The listing builds one solid part. Answer for the finished solid, in the listing's coordinates (mm). A direction names the side the tool comes from. Give positions to 0.01 mm unless a question says otherwise; leave off trailing zeros. Write each loop counter-clockwise with the first axis right and the second up, starting at its lowest first coordinate (ties: lowest second). Pieces come first, ordered by that corner, then holes. Notation, with made-up numbers: (17.25, -24.5) -> (48.25, -24.5) arc R18 cw to (48.25, -19.5) -> close; hole circle Ø9 at (77, 41). An arc over 180 degrees is marked (long way). Write each question's results on one line, items separated by ' | '. Start each with the question number.
from build123d import *

# Parameters (mm, degrees)
SKETCH1_W            = 10
SKETCH1_H            = 10
BOSS_EXTRUDE1_DEPTH  = 10
SKETCH2_W            = 10
SKETCH2_H            = 5
BOSS_EXTRUDE2_DEPTH  = 35
SKETCH3_R            = 1.25
CUT_EXTRUDE1_DEPTH   = 5
FILLET1_R            = 5
SKETCH4_W            = 6
SKETCH4_H            = 2
CUT_EXTRUDE2_DEPTH   = 20
SKETCH6_W            = 1.5
SKETCH6_H            = 5
CUT_EXTRUDE3_DEPTH   = 2
CUT_EXTRUDE4_DEPTH   = 10
LPATTERN1_COUNT      = 9
LPATTERN1_PITCH      = 4
LPATTERN1_COUNT_DIR2 = 2
LPATTERN1_PITCH_DIR2 = 8


with BuildPart() as part:
    # Sketch1 → Boss-Extrude1 (new body, symmetric)
    with BuildSketch(Plane(origin=(0, 0, 0), x_dir=(1, 0, 0), z_dir=(0, 1, 0))):
        Rectangle(SKETCH1_W, SKETCH1_H)
    extrude(amount=BOSS_EXTRUDE1_DEPTH, both=True)

    # Sketch2 → Boss-Extrude2 (add)
    with BuildSketch(Plane.XY.offset(5)):
        Rectangle(SKETCH2_W, SKETCH2_H)
    extrude(amount=BOSS_EXTRUDE2_DEPTH)

    # Sketch3 → Cut-Extrude1 (cut)
    with BuildSketch(Plane(origin=(0, 2.5, 0), x_dir=(1, 0, 0), z_dir=(0, 1, 0))):
        with Locations((0, -17)):
            Circle(SKETCH3_R)
    extrude(amount=-CUT_EXTRUDE1_DEPTH, mode=Mode.SUBTRACT)

    # Fillet1
    fillet1_edges = [part.edges().sort_by_distance(p)[0] for p in [
        (-5, 0, 40),
        (5, 0, -5),
    ]]
    fillet(fillet1_edges, radius=FILLET1_R)

    # Sketch4 → Cut-Extrude2 (cut)
    with BuildSketch(Plane(origin=(0, 10, 0), x_dir=(1, 0, 0), z_dir=(0, 1, 0))):
        with Locations((2, 0)):
            Rectangle(SKETCH4_W, SKETCH4_H)
    extrude(amount=-CUT_EXTRUDE2_DEPTH, mode=Mode.SUBTRACT)

    # Sketch6 → Cut-Extrude3 (cut)
    with BuildSketch(Plane.ZY.offset(5)):
        with Locations((5.75, 0)):
            Rectangle(SKETCH6_W, SKETCH6_H)
    cut_extrude3 = extrude(amount=-CUT_EXTRUDE3_DEPTH, mode=Mode.SUBTRACT)

    # Sketch7 → Cut-Extrude4 (cut)
    with BuildSketch(Plane(origin=(-1, 0, 0), x_dir=(0, 0, -1), z_dir=(1, 0, 0))):
        Polygon((-1, 5), (11.1033346, -5.155903599), (9.817759381, -6.687992485), (-1, 2.389185421), align=None)
    extrude(amount=CUT_EXTRUDE4_DEPTH, mode=Mode.SUBTRACT)

    # LPattern1: Cut-Extrude3 9 × 2, 12 skipped
    with Locations(*[(j * LPATTERN1_PITCH_DIR2, 0, i * LPATTERN1_PITCH) for i in range(LPATTERN1_COUNT) for j in range(LPATTERN1_COUNT_DIR2) if (i, j) not in ((0, 0), (0, 1), (1, 0), (1, 1), (2, 0), (2, 1), (3, 0), (3, 1), (4, 0), (5, 0), (6, 0), (7, 0), (8, 0))]):
        add(cut_extrude3, mode=Mode.SUBTRACT)


solid = part.part
1. Section D-D (x = 0.75) is taken. Write down the section's boundary in (y, z).
2. Section A-A (x = -4) is taken. Write down the section's boundary in (y, z), then the cut area to 4 significant figures.
3. Section C-C (y = 8.25) is taken. Write down the section's boundary in (x, z), then the cut area to 3 significant figures.
4. Consider probe 1 along X at (y, z) = (-0.6, 17); probe 2 along Z at (x, y) = (0, -1.1); probe 3 along Z at (x, y) = (0, -0.8). Determine where each line is inside the solid, lowest interval first. Write a range as [from, to].
5. The mould has two halves that part along Z. Classify faces 6 (the flat face through (0, -2.5, 22)), 7 (the flat face through (4, 0, 21)), 8 (the cylindrical face through (3, -6, -4)): pulls with the +Z half, pulls with the -Z half, needs draft (parallel to the pull), parting line crosses it, or undercut.
6. Each of these flat-tipped pins is pushed along its axis until it touches: pin 1 Ø0.6 at (x, y) = (4, -0.5) entering from -Z; pin 2 Ø5 at (x, z) = (2, 22.5) entering from +Y; pin 3 Ø1 at (x, y) = (4, -1) entering from -Z. Where does it stop, or does it pass through?
7. A tool of negligible diameter and unlimited length cuts with its end or side. For faces 1 (the flat face through (5, 0, 36)), 2 (the flat face through (0, 2.5, 22)), 3 (the flat face through (1.253, -0.618, -2.584)), 4 (the flat face through (4, 0, 26.5)), 5 (the flat face through (-3, 0, 6)), from which of +Z, -Z, +X, -X, +Y, -Y can it reach the whole face along a straight path? Write none if from no direction.
8. Section B-B (z = 17) is taken. Write down the section's boundary in (x, y).
Results:
1) outline: (-10, -4.94) -> (-2.6, -4.94) -> (0.71, -1) -> (-10, -1) -> close; (-10, 1) -> (10, 1) -> (10, 5) -> (2.5, 5) -> (2.5, 16) -> (-2.5, 16) -> (-2.5, 5) -> (-10, 5) -> close; (-2.5, 18) -> (2.5, 18) -> (2.5, 40) -> (-2.5, 40) -> close; (0.01, -4.94) -> (10, -4.94) -> (10, -1) -> (3.32, -1) -> close
2) outline: (-10, -5) -> (10, -5) -> (10, 5) -> (-10, 5) -> close; (-2.5, 6.5) -> (2.5, 6.5) -> (2.5, 38) -> (-2.5, 38) -> close | area: 357.5 mm²
3) outline: (-5, -5) -> (0, -5) arc R5 ccw to (4.9, -1) -> (-1, -1) -> (-1, 1) -> (5, 1) -> (5, 5) -> (-5, 5) -> close | area: 82.7 mm²
4) probe 1: x = [-5, -1.25], [1.25, 5] | probe 2: z = [-3.16, -1], [1, 15.75], [18.25, 40] | probe 3: z = [-2.8, -1], [1, 15.75], [18.25, 40]
5) face 6: needs draft | face 7: undercut | face 8: pulls with the -Z half
6) pin 1: stops at z = -2.8 | pin 2: stops at y = 2.5 | pin 3: stops at z = -3.44
7) face 1: +Z, -Z, +X, +Y, -Y | face 2: +Z, +X, -X, +Y | face 3: +X | face 4: +X, +Y, -Y | face 5: -X, +Y, -Y
8) outline: (-5, -2.5) -> (-1.25, -2.5) -> (-1.25, 2.5) -> (-5, 2.5) -> close; (1.25, -2.5) -> (5, -2.5) -> (5, 2.5) -> (1.25, 2.5) -> close
